Work out the finished part from the listing and answer in its coordinate system (mm). A direction names the side the tool comes from. Coordinates: 2 decimals unless noted, no trailing zeros. Order: outer loops, then holes, each group sorted by start corner. A loop starts at its lowest first (then second) coordinate and runs counter-clockwise, first axis right, second up.
1. The part is cut by section C-C, the plane z = 40.5. Give the vertices of the cut face in (x, y), then the cut area to 3 significant figures.
2. The part is cut by section A-A, the plane x = 0. Give the vertices of the cut face in (y, z), then the cut area to 3 significant figures.
3. The part is cut by section D-D, the plane y = -32.5. Give the vertices of the cut face in (x, z).
4. A flat-ended cylindrical pin translates along its axis: pin 1 Ø1.5 at (y, z) = (-0.5, 33.5) entering from +X. Find the tip coordinate at first contact, or state that the pin passes through.
5. A tool of negligible diameter and unlimited length cuts with its end or side. For faces 1 (the flat face through (-17, -9, 25.4)), 2 (the flat face through (25.4, -1, -26)), from which of +Z, -Z, +X, -X, +Y, -Y can it reach the whole face along a straight path? Write none if from no direction.
6. The part is cut by section B-B, the plane y = 0. Give the vertices of the cut face in (x, z), then the cut area to 3 significant figures.
7. Find the intervals of material crossed by probe 1 along Z at (x, y) = (-22, -16.5); probe 2 along Y at (x, z) = (-1, 38); probe 3 along X at (y, z) = (3, 41), in increasing order.
```python
from build123d import *

# Parameters (mm, degrees)
F0_W     = 50.8
F0_H     = 101.6
F1_DEPTH = 38.1
F2_R     = 19.05
F3_DEPTH = 25.4


with BuildPart() as f1:
    # F0 (on Front) → F1 (new body, symmetric)
    with BuildSketch(Plane.XZ):
        with Locations((0, -25.4)):
            Rectangle(F0_W, F0_H)
    extrude(amount=F1_DEPTH, both=True)

    # F2 (on face) → F3 (join)
    with BuildSketch(Plane.XY.offset(25.4)):
        Circle(F2_R)
    extrude(amount=F3_DEPTH)


solid = f1.part
```
Geometry says:
1. outline: circle Ø38.1 at (0, 0)
1. area: 1,140 mm2
2. outline: (-38.1, -76.2) - (38.1, -76.2) - (38.1, 25.4) - (19.05, 25.4) - (19.05, 50.8) - (-19.05, 50.8) - (-19.05, 25.4) - (-38.1, 25.4) - close
2. area: 8,710 mm2
3. outline: (-25.4, -76.2) - (25.4, -76.2) - (25.4, 25.4) - (-25.4, 25.4) - close
4. pin 1: stops at x = 19.05
5. face 1: +Z
5. face 2: +Z, -Z, +X, +Y, -Y
6. outline: (-25.4, -76.2) - (25.4, -76.2) - (25.4, 25.4) - (19.05, 25.4) - (19.05, 50.8) - (-19.05, 50.8) - (-19.05, 25.4) - (-25.4, 25.4) - close
6. area: 6,130 mm2
7. probe 1: z = -76.2 to 25.4
7. probe 2: y = -19.02 to 19.02
7. probe 3: x = -18.81 to 18.81
